```python
from build123d import *

# Parameters (mm, degrees)
SALIENTE_EXTRUIR1_DEPTH = 3.2
CROQUIS3_R              = 2.05
CORTAR_EXTRUIR2_DEPTH   = 3.2
CORTAR_EXTRUIR3_DEPTH   = 3.2
CORTAR_EXTRUIR4_DEPTH   = 3.2
REDONDEO1_R             = 3
CROQUIS6_R              = 1.55
CORTAR_EXTRUIR5_DEPTH   = 3.2


with BuildPart() as part:
    # Croquis1 → Saliente-Extruir1 (new body)
    with BuildSketch(Plane(origin=(0, 0, 0), x_dir=(1, 0, 0), z_dir=(0, 1, 0))):
        Polygon((7, 66.1), (10, 66.1), (10, 62.9), (7, 62.9), (7, 61.5), (3, 61.5), (3, 62.9), (0, 62.9), (0, 57), (-3, 57), (-3, 51), (0, 51), (0, 0), (165, 0), (165, 1.5), (168, 1.5), (168, 7.5), (165, 7.5), (165, 13.4), (162, 13.4), (162, 12), (158, 12), (158, 13.4), (155, 13.4), (155, 16.6), (158, 16.6), (158, 18), (162, 18), (162, 16.6), (165, 16.6), (165, 22.5), (168, 22.5), (168, 28.5), (165, 28.5), (165, 570), (30, 570), (30, 566.9), (21.6, 566.9), (21.6, 563.9), (23, 563.9), (23, 559.9), (21.6, 559.9), (21.6, 556.9), (18.4, 556.9), (18.4, 559.9), (17, 559.9), (17, 563.9), (18.4, 563.9), (18.4, 566.9), (10, 566.9), (10, 570), (0, 570), (0, 543), (-3, 543), (-3, 537), (0, 537), (0, 531.1), (3, 531.1), (3, 532.5), (7, 532.5), (7, 531.1), (10, 531.1), (10, 527.9), (7, 527.9), (7, 526.5), (3, 526.5), (3, 527.9), (0, 527.9), (0, 522), (-3, 522), (-3, 516), (0, 516), (0, 388), (-3, 388), (-3, 382), (0, 382), (0, 376.1), (3, 376.1), (3, 377.5), (7, 377.5), (7, 376.1), (10, 376.1), (10, 372.9), (7, 372.9), (7, 371.5), (3, 371.5), (3, 372.9), (0, 372.9), (0, 367), (-3, 367), (-3, 361), (0, 361), (0, 233), (-3, 233), (-3, 227), (0, 227), (0, 221.1), (3, 221.1), (3, 222.5), (7, 222.5), (7, 221.1), (10, 221.1), (10, 217.9), (7, 217.9), (7, 216.5), (3, 216.5), (3, 217.9), (0, 217.9), (0, 212), (-3, 212), (-3, 206), (0, 206), (0, 78), (-3, 78), (-3, 72), (0, 72), (0, 66.1), (3, 66.1), (3, 67.5), (7, 67.5), align=None)
    extrude(amount=SALIENTE_EXTRUIR1_DEPTH)

    # Croquis3 → Cortar-Extruir2 (cut)
    with BuildSketch(Plane(origin=(0, 3.2, 0), x_dir=(1, 0, 0), z_dir=(0, 1, 0))):
        with Locations((40, 80)):
            Circle(CROQUIS3_R)
        with Locations((90, 80)):
            Circle(CROQUIS3_R)
        with Locations((40, 230)):
            Circle(CROQUIS3_R)
    extrude(amount=-CORTAR_EXTRUIR2_DEPTH, mode=Mode.SUBTRACT)

    # Croquis4 → Cortar-Extruir3 (cut)
    with BuildSketch(Plane.XZ):
        with BuildLine():
            Line((143, -30.5), (129, -30.5))
            ThreePointArc((129, -30.5), (127.585786438, -31.085786438), (127, -32.5))
            Line((127, -32.5), (127, -38.5))
            ThreePointArc((127, -38.5), (127.585786438, -39.914213562), (129, -40.5))
            Line((129, -40.5), (143, -40.5))
            ThreePointArc((143, -40.5), (144.414213562, -39.914213562), (145, -38.5))
            Line((145, -38.5), (145, -32.5))
            ThreePointArc((145, -32.5), (144.414213562, -31.085786438), (143, -30.5))
        make_face()
    extrude(amount=-CORTAR_EXTRUIR3_DEPTH, mode=Mode.SUBTRACT)

    # Croquis5 → Cortar-Extruir4 (cut)
    with BuildSketch(Plane.XZ):
        with BuildLine():
            Line((35, -570), (165, -570))
            Line((165, -570), (165, -31.5))
            ThreePointArc((165, -31.5), (70.982951471, -293.744955787), (35, -570))
        make_face()
    extrude(amount=-CORTAR_EXTRUIR4_DEPTH, mode=Mode.SUBTRACT)

    # Redondeo1
    redondeo1_edges = [part.edges().sort_by_distance(p)[0] for p in [
        (35, 1.6, -570),
    ]]
    fillet(redondeo1_edges, radius=REDONDEO1_R)

    # Croquis6 → Cortar-Extruir5 (cut)
    with BuildSketch(Plane.XZ):
        with Locations((110, -95)):
            Circle(CROQUIS6_R)
        with Locations((35, -95)):
            Circle(CROQUIS6_R)
        with Locations((60, -175)):
            Circle(CROQUIS6_R)
        with Locations((15, -175)):
            Circle(CROQUIS6_R)
        with Locations((77, -35.5)):
            Circle(CROQUIS6_R)
        with Locations((37, -215.5)):
            Circle(CROQUIS6_R)
        with Locations((57, -155.5)):
            Circle(CROQUIS6_R)
    extrude(amount=-CORTAR_EXTRUIR5_DEPTH, mode=Mode.SUBTRACT)


solid = part.part
```
Design review of the part built by this model. Coordinates are the model's own, in mm. Round coordinates to 2 decimals unless told otherwise and drop trailing zeros. Write each loop counter-clockwise with the first axis right and the second up, starting at its lowest first coordinate (ties: lowest second). Pieces come first, ordered by that corner, then holes. Notation, with made-up numbers: (-36.75, -26.5) -> (-31.75, -26.5) arc R29 cw to (-31.75, -4.5) -> close; hole circle Ø4 at (-10, 32.5). An arc over 180 degrees is marked (long way). Answer in a Markdown table with one row per item.
Q1. Clearance check with flat-ended pins moving along their axes: pin 1 Ø1.5 at (x, y) = (-2, 2) entering from -Z; pin 2 Ø1 at (y, z) = (1, -379) entering from -X; pin 3 Ø0.7 at (y, z) = (1.5, -376.5) entering from +X. State where each tip first meets the part, or that it passes through.
The answers:
| item | result |
|---|---|
| pin 1 | z = -543 |
| pin 2 | x = 0 |
| pin 3 | x = 53.89 |
Q2. Take a section at A-A, the plane y = 2.4. Count the separate pieces of the cut face and the enclosed holes in it, then the cut area to 3 significant figures.
The answers:
| item | result |
|---|---|
| separate pieces | 1 |
| enclosed holes | 11 |
| area | 47,600 mm² |
Q3. To check wall thickness, follow L1, parallel to X at y = 2.05, z = -175; L2, parallel to X at y = 0.75, z = -215.5; L3, parallel to X at y = 2.1, z = -230. State the ranges of each line that lie inside material, in increasing order. Write a range as [from, to].
The answers:
| item | result |
|---|---|
| L1 | [0, 13.45], [16.55, 58.45], [61.55, 105.71] |
| L2 | [0, 35.45], [38.55, 92.48] |
| L3 | [-3, 37.95], [42.05, 88.1] |
Q4. Take a section at B-B, the plane z = -267.5. State the section outline as (x, y) points.
The answers:
| item | result |
|---|---|
| outline | (0, 0) -> (77.61, 0) -> (77.61, 3.2) -> (0, 3.2) -> close |
Q5. Take a section at C-C, the plane z = -444.5. State the section outline as (x, y) points, then the cut area to 3 significant figures.
The answers:
| item | result |
|---|---|
| outline | (0, 0) -> (43.87, 0) -> (43.87, 3.2) -> (0, 3.2) -> close |
| area | 140 mm² |
